Autodesk Inventor part; units mm, degrees
ref_plane "YZ Plane" through (0, 0, 0) normal (1, 0, 0) x (0, 1, 0)
ref_plane "XZ Plane" through (0, 0, 0) normal (0, 1, 0) x (-1, 0, 0)
ref_plane "XY Plane" through (0, 0, 0) normal (0, 0, 1) x (1, 0, 0)
sketch "Sketch1" plane through (0, 0, 0) normal (0, 1, 0) x (-1, 0, 0)
  line L0 (0, 0) -> (0, -7.35)
  line L1 (0, -7.35) -> (20, -7.35)
  line L2 (0, 0) -> (20, 0)
  line L3 (0, 0) -> (0, -3.68)
  line L4 (0, -3.68) -> (4.5, -3.68) construction
  line L5 (4.5, -3.68) -> (14, -3.68) construction
  line L6 (14, -3.68) -> (22, -3.68) construction
  line L7 (22, -3.68) -> (25, -3.68) construction
  line L8 (25, -3.68) -> (28, -3.68) construction
  line L9 (28, -3.68) -> (28.5, -3.68) construction
  arc A0 (28.8344, -6.1575) -> (28.8372, -1.2028) centre (28.5, -3.68) ccw
  circle A1 centre (28, -3.68) radius 0.67
  circle A2 centre (25, -3.68) radius 0.67
  circle A3 centre (22, -3.68) radius 0.67
  line L10 (20, 0) -> (28.8372, -1.2028)
  line L11 (20, -7.35) -> (28.8344, -6.1575)
  arc A4 (4.5, -2.255) -> (4.5, -5.105) centre (4.5, -3.68) ccw
  arc A5 (14, -5.105) -> (14, -2.255) centre (14, -3.68) ccw
  line L12 (14, -2.255) -> (4.5, -2.255)
  line L13 (4.5, -5.105) -> (14, -5.105)
  dimension "d0" = 7.35
  dimension "d1" = 20
  dimension "d2" = 20
  dimension "d3" = 3.68
  dimension "d4" = 4.5
  dimension "d5" = 9.5
  dimension "d6" = 8
  dimension "d7" = 3
  dimension "d8" = 3
  dimension "d9" = 0.5
  dimension "d10" = 5
  dimension "d11" = 1.34
  dimension "d12" = 1.34
  dimension "d13" = 1.34
  dimension "d16" = 2.85
  dimension "d17" = 2.85
extrude "Extrusion1" add sketch "Sketch1" along normal blind 2
properties part number "MMAE 232 CAD Assignment 2 Servo Horn 1-Nicholas Skiba"
Could you check a few things on this model? Use its own coordinates, in mm. A direction names the side the tool comes from. Give positions to 0.01 mm unless a question says otherwise; leave off trailing zeros. Loops run counter-clockwise (first coordinate to the right, second up) from the corner with the lowest first, then second, coordinate; pieces in that order, holes last. Notation, with made-up numbers: (-38.5, 87.5) -> (15.5, 87.5) arc R31 cw to (15.5, 118.5) -> close; hole circle Ø3 at (3.5, 52.25). An arc over 180 degrees is marked (long way). Return JSON: item names as keys, results as strings.
Item 1: I'm going to push a flat-ended pin straight in: pin 1 (1.5 mm diameter, centred on x = -6, z = -4.5, fed in from -Y). Where does the tip first touch, or does it pass through?
Geometry results:
{"pin 1": "stops at y = 0"}
Item 2: I need wall thicknesses on L1, parallel to X at y = 1.8, z = -3.5; L2, parallel to Z at x = -9.5, y = 0.2 (3 decimals); L3, parallel to X at y = 1.45, z = -3.25. Which ranges of each line are inside material? Lowest first, please. Write a range as from..to.
Geometry results:
{"L1": "x = -30.99..-28.65, -27.35..-25.65, -24.35..-22.65, -21.35..-15.41, -3.09..0", "L2": "z = -7.35..-5.105, -2.255..0", "L3": "x = -30.96..-28.51, -27.49..-25.51, -24.49..-22.51, -21.49..-15.36, -3.14..0"}
Item 3: If we section it at A-A on x = -12.5: List the corners of the cut face in (y, z) for me (3 decimals), plus the area to 3 significant figures.
Geometry results:
{"outline": "(0, -7.35) -> (2, -7.35) -> (2, -5.105) -> (0, -5.105) -> close; (0, -2.255) -> (2, -2.255) -> (2, 0) -> (0, 0) -> close", "area": "9.00 mm²"}
Item 4: If we section it at D-D on x = -22: List the corners of the cut face in (y, z) for me, plus the area to 3 significant figures.
Geometry results:
{"outline": "(0, -7.08) -> (2, -7.08) -> (2, -4.35) -> (0, -4.35) -> close; (0, -3.01) -> (2, -3.01) -> (2, -0.27) -> (0, -0.27) -> close", "area": "10.9 mm²"}
Item 5: Which directions (+Z, -Z, +X, -X, +Y, -Y) give clear straight access to the entire face, cutting with the end or side of a thin tool? Please do faces 4 (the cylindrical face through (-15.425, 0.986, -3.649)), 5 (the flat face through (-15, 2, -5)).
Geometry results:
{"face 4": "+Y, -Y", "face 5": "+Z, -Z, +X, -X, +Y"}
Item 6: If we section it at C-C on y = 0.8: Count the separate pieces of the cut face and the enclosed holes in it, plus the area to 3 significant figures.
Geometry results:
{"separate pieces": "1", "enclosed holes": "4", "area": "172 mm²"}
Item 7: We'd pull the mould along X, two halves only. Please class faces 1 (the flat face through (-9, 1, -5.105)), 2 (the flat face through (-24.4, 1, -0.6)), 3 (the flat face through (-10, 1, 0)): +X half, -X half, draft (parallel to the pull), parting line (faces both ways), or undercut.
Geometry results:
{"face 1": "undercut", "face 2": "-X half", "face 3": "draft"}
Item 8: If we section it at B-B on z = -3.68: List the corners of the cut face in (x, y) for me (3 decimals).
Geometry results:
{"outline": "(-31, 0) -> (-28.67, 0) -> (-28.67, 2) -> (-31, 2) -> close; (-27.33, 0) -> (-25.67, 0) -> (-25.67, 2) -> (-27.33, 2) -> close; (-24.33, 0) -> (-22.67, 0) -> (-22.67, 2) -> (-24.33, 2) -> close; (-21.33, 0) -> (-15.425, 0) -> (-15.425, 2) -> (-21.33, 2) -> close; (-3.075, 0) -> (0, 0) -> (0, 2) -> (-3.075, 2) -> close"}
